from build123d import *

# Parameters (mm, degrees)
SKETCH1_W                                       = 44
SKETCH1_H                                       = 6
EXTRUDE1_DEPTH                                  = 27
CSK_FOR_M6_FLAT_HEAD_MACHINE_SCREW1_D           = 5
CSK_FOR_M6_FLAT_HEAD_MACHINE_SCREW1_CSINK_D     = 10
CSK_FOR_M6_FLAT_HEAD_MACHINE_SCREW1_CSINK_ANGLE = 90


with BuildPart() as part:
    # Sketch1 → Extrude1 (new, symmetric)
    with BuildSketch(Plane.XY):
        with Locations((22, 3)):
            Rectangle(SKETCH1_W, SKETCH1_H)
    extrude(amount=EXTRUDE1_DEPTH, both=True)

    # CSK for M6 Flat Head Machine Screw1 (through all)
    with Locations(Plane(origin=(10, 6, 0), x_dir=(0, 0, 1), z_dir=(0, 1, 0))):
        with Locations((0, 0), (0, 24)):
            CounterSinkHole(CSK_FOR_M6_FLAT_HEAD_MACHINE_SCREW1_D / 2, CSK_FOR_M6_FLAT_HEAD_MACHINE_SCREW1_CSINK_D / 2, counter_sink_angle=CSK_FOR_M6_FLAT_HEAD_MACHINE_SCREW1_CSINK_ANGLE)


solid = part.part
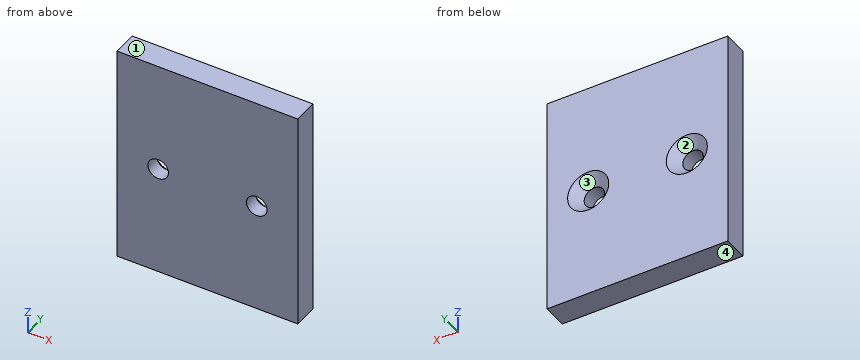
Can you work these out from the model? Positions are in its coordinate system, mm. Face numbers are marked on the shaded views. Round coordinates to 2 decimals unless told otherwise and drop trailing zeros. Loops run counter-clockwise (first coordinate to the right, second up) from the corner with the lowest first, then second, coordinate; pieces in that order, holes last. Notation, with made-up numbers: (-21.75, 44) - (-3.75, 44) arc R18 cw to (-3.75, 63) - close; hole circle Ø2 at (26.5, 48.5). An arc over 180 degrees is marked (long way). Use CSV: the item, a comma, the result in double quotes. Start each with the question number.
1) If we section it at B-B on y = 1.7: Write out the boundary of the cut face in (x, z), plus the area to 3 significant figures.
2) For pin 1 Ø5 at (x, z) = (27.5, -12) entering from -Y, with a flat end and sliding along its axis, tell me the tip position at first contact or that it passes through.
3) If we section it at D-D on y = 5.05: Write out the boundary of the cut face in (x, z), plus the area to 3 significant figures.
4) Please list where these lines run through material, in increasing order: probe 1 along X at (y, z) = (1.6, 0); probe 2 along Z at (x, y) = (34, 1.15); probe 3 along Z at (x, y) = (37, 4.75). Write a range as [from, to].
5) If we section it at A-A on z = 0: Write out the boundary of the cut face in (x, y).
6) We'd pull the mould along Z, two halves only. Please class the marked faces 1, 2, 3 and 4: released by +Z, released by -Z, zero draft, split by the parting line, or undercut.
7) If we section it at C-C on x = 34: Write out the boundary of the cut face in (y, z).
Geometry results:
1,outline,"(0, -27) - (44, -27) - (44, 27) - (0, 27) - close; hole circle Ø5 at (10, 0); hole circle Ø5 at (34, 0)"
1,area,"2,340 mm2"
2,pin 1,"stops at y = 0"
3,outline,"(0, -27) - (44, -27) - (44, 27) - (0, 27) - close; hole circle Ø8.1 at (10, 0); hole circle Ø8.1 at (34, 0)"
3,area,"2,270 mm2"
4,probe 1,"x = [0, 7.5], [12.5, 31.5], [36.5, 44]"
4,probe 2,"z = [-27, -2.5], [2.5, 27]"
4,probe 3,"z = [-27, -2.25], [2.25, 27]"
5,outline,"(0, 0) - (7.5, 0) - (7.5, 3.5) - (5, 6) - (0, 6) - close; (12.5, 0) - (31.5, 0) - (31.5, 3.5) - (29, 6) - (15, 6) - (12.5, 3.5) - close; (36.5, 0) - (44, 0) - (44, 6) - (39, 6) - (36.5, 3.5) - close"
6,face 1,"released by +Z"
6,face 2,"undercut"
6,face 3,"undercut"
6,face 4,"released by -Z"
7,outline,"(0, -27) - (6, -27) - (6, -5) - (3.5, -2.5) - (0, -2.5) - close; (0, 2.5) - (3.5, 2.5) - (6, 5) - (6, 27) - (0, 27) - close"
